Here's how the part is built. I have some questions about the finished solid (model axes, mm). Face numbers are marked on the shaded views. A direction names the side the tool comes from. Coordinates: 2 decimals unless noted, no trailing zeros. Write each loop counter-clockwise with the first axis right and the second up, starting at its lowest first coordinate (ties: lowest second). Pieces come first, ordered by that corner, then holes. Notation, with made-up numbers: (-28, 2) -> (15, 2) arc R19 cw to (15, 14) -> close; hole circle Ø7 at (55.5, 15). An arc over 180 degrees is marked (long way). Put each result on its own line as item: value. Start each with the question number.
Item 1: I want a section at A-A, the plane x = 64. List the corners of the cut face in (y, z) for me, then the cut area to 3 significant figures.
Item 2: I need wall thicknesses on line 1 (Y direction, x = 77, z = 0.5); line 2 (X direction, y = -13, z = -3); line 3 (X direction, y = 24, z = -5.5). Which ranges of each line are inside material? Lowest first, please. Write a range as [from, to].
Item 3: On a 3-axis mill with a long thin cutter (end or side, diameter ignored), from which of +Z, -Z, +X, -X, +Y, -Y can I reach the whole of each face in a straight line? I mean the marked faces 1 and 2. Say none if no direction works.
Item 4: For pin 1 (10 mm diameter, centred on y = 18.5, z = -11.5, fed in from +X); pin 2 (4 mm diameter, centred on y = 16.5, z = 12, fed in from +X); pin 3 (3 mm diameter, centred on x = 39, z = 1.5, fed in from -Y); pin 4 (11.5 mm diameter, centred on y = 17, z = -1, fed in from -X), each with a flat end and sliding along its axis, tell me the tip position at first contact or that it passes through.
Item 5: If we mould it in two halves opening along X, with no side actions, what happens to the marked faces 3, 4 and 5? For each: released by +X, released by -X, zero draft, split by the parting line, or undercut.
from build123d import *
from build123d.topology import SkipClean

# Parameters (mm, degrees)
SKETCH5_W          = 2
SKETCH5_H          = 25
SKETCH2_R          = 3
CUT_EXTRUDE1_DEPTH = 6
FILLET1_R          = 2
CUT_EXTRUDE2_DEPTH = 6
FILLET2_R          = 0.5
CUT_EXTRUDE3_REACH = 132.8


with BuildPart() as part:
    # Sketch1 → Revolve1 (revolve)
    with BuildSketch(Plane.XY, mode=Mode.PRIVATE) as revolve1_sk:
        Polygon((130.8, 11.45), (0, 11.45), (0, 26), (6, 26), (6, 12.9), (10, 12.9), (10, 15.5), (12, 15.5), (12, 14), (13, 14), (13.5, 22.5), (16, 22.5), (17, 12.9), (21.4, 12.9), (21.4, 14.75), (23, 14.75), (23, 12.65), (130.8, 12.65), align=None)
    revolve(revolve1_sk.sketch.rotate(Axis((0, 0, 0), (1, 0, 0)), 90), axis=Axis((0, 0, 0), (1, 0, 0)))  # turned: the seam where the file's is

    # Sketch5 → Cut-Revolve1 (revolve, cut)
    with BuildSketch(Plane.XY, mode=Mode.PRIVATE) as cut_revolve1_sk:
        with Locations((3, 32.5)):
            Rectangle(SKETCH5_W, SKETCH5_H)
    revolve(cut_revolve1_sk.sketch.rotate(Axis((0, 0, 0), (-1, 0, 0)), 270), axis=Axis((0, 0, 0), (-1, 0, 0)), mode=Mode.SUBTRACT)  # turned: the seam where the file's is

    # Sketch2 → Cut-Extrude1 (cut)
    with SkipClean():  # keep this step's faces unmerged: merging them makes the solid invalid here
        with BuildSketch(Plane.ZY):
            with Locations((-5.176381, 19.318517)):
                Circle(SKETCH2_R)
            with Locations((6.840403, 18.793852)):
                Circle(SKETCH2_R)
            with BuildLine():
                Line((14.627074, 13.639967), (16, 20.493902))
                ThreePointArc((16, 20.493902), (0, -26), (-16, 20.493902))
                Line((-16, 20.493902), (-15.760215, 12.31323))
                ThreePointArc((-15.760215, 12.31323), (0.872388, -19.980964), (14.627074, 13.639967))
            make_face()
        extrude(amount=-CUT_EXTRUDE1_DEPTH, mode=Mode.SUBTRACT)

    # Fillet1
    fillet1_edges = [part.edges().sort_by_distance(p)[0] for p in [
        (1, 12.31323, -15.760215),
        (5, 12.31323, -15.760215),
        (1, 13.639967, 14.627074),
        (5, 13.639967, 14.627074),
    ]]
    fillet(fillet1_edges, radius=FILLET1_R)

    # Sketch3 → Cut-Extrude2 (cut)
    with SkipClean():  # keep this step's faces unmerged: merging them makes the solid invalid here
        with BuildSketch(Plane.ZY):
            with BuildLine():
                Line((-16.968292, -1.037825), (-19.995549, -0.421923))
                ThreePointArc((-19.995549, -0.421923), (-12.586408, -15.542919), (3.744606, -19.646321))
                Line((3.744606, -19.646321), (2.51276, -16.81327))
                ThreePointArc((2.51276, -16.81327), (-10.698447, -13.211481), (-16.968292, -1.037825))
            make_face()
        extrude(amount=-CUT_EXTRUDE2_DEPTH, mode=Mode.SUBTRACT)

    # Fillet2
    fillet2_edges = [part.edges().sort_by_distance(p)[0] for p in [
        (3, -19.646321, 3.744606),
        (3, -0.421923, -19.995549),
        (1, 20.493902, 16),
        (5, 20.493902, 16),
        (1, 20.493902, -16),
        (5, 20.493902, -16),
    ]]
    fillet(fillet2_edges, radius=FILLET2_R)

    # Sketch4 → Cut-Extrude3 (cut, up to next)
    with BuildSketch(Plane.ZY, mode=Mode.PRIVATE) as cut_extrude3_sk1:
        Polygon((-5.843402, 18.975614), (-4.509359, 19.661419), (-10.480395, 35.216499), (-11.814438, 34.530693), align=None)
    cut_extrude3_tool1 = extrude(cut_extrude3_sk1.sketch, amount=-CUT_EXTRUDE3_REACH, mode=Mode.PRIVATE) & part.part
    add(cut_extrude3_tool1.solids().sort_by_distance((0, 27.096056, -8.161899))[0], mode=Mode.SUBTRACT)
    # Sketch4 → Cut-Extrude3 (cut, up to next)
    with BuildSketch(Plane.ZY, mode=Mode.PRIVATE) as cut_extrude3_sk2:
        Polygon((6.108448, 18.957382), (7.572358, 18.630323), (10.539953, 35.460393), (9.076043, 35.787451), align=None)
    cut_extrude3_tool2 = extrude(cut_extrude3_sk2.sketch, amount=-CUT_EXTRUDE3_REACH, mode=Mode.PRIVATE) & part.part
    add(cut_extrude3_tool2.solids().sort_by_distance((0, 27.208887, 8.324201))[0], mode=Mode.SUBTRACT)


solid = part.part
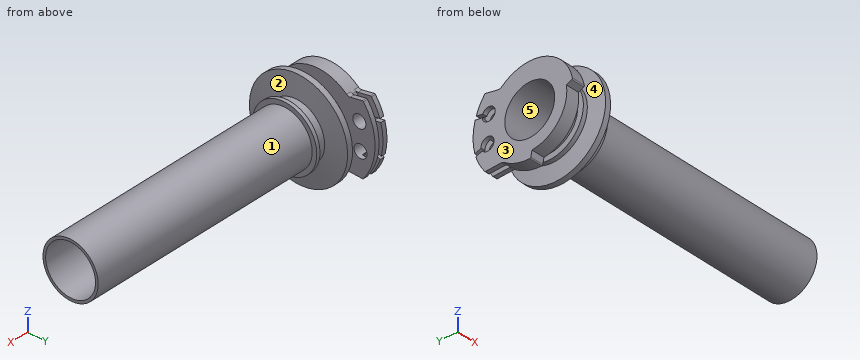
Calculated:
1. outline: circle Ø25.3 at (0, 0); hole circle Ø22.9 at (0, 0)
1. area: 90.9 mm2
2. line 1: y = [-12.64, -11.44], [11.44, 12.64]
2. line 2: x = [0, 6], [10, 16.95], [21.4, 23]
2. line 3: x = [0, 2], [4, 6]
3. face 1: +X
3. face 2: none
4. pin 1: stops at x = 16.6
4. pin 2: stops at x = 16.43
4. pin 3: stops at y = -12.65
4. pin 4: stops at x = 0
5. face 3: released by -X
5. face 4: undercut
5. face 5: zero draft
